Input: part model. Units: mm. Frame: model coordinates. Face numbers are marked on the shaded views. A direction names the side the tool comes from. Coordinates: 2 decimals unless noted, no trailing zeros. Write each loop counter-clockwise with the first axis right and the second up, starting at its lowest first coordinate (ties: lowest second). Pieces come first, ordered by that corner, then holes. Notation, with made-up numbers: M 50.5,26 L 70.5,26 A28 cw 70.5,48 Z; hole C 26,33 d9. An arc over 180 degrees is marked long. Use CSV: the item, a comma, the result in double quotes.
```python
from build123d import *

# Parameters (mm, degrees)
SKETCH_2_W          = 80
SKETCH_2_H          = 82
EXTRUDE_2_DEPTH     = 30
SKETCH_3_R          = 12
CUT_EXTRUDE_1_DEPTH = 65.660652641
CUT_EXTRUDE_2_DEPTH = 65.660652641
HOLE_WIZARD_M4_1_D  = 3.3
HOLE_WIZARD_M4_2_D  = 3.3


with BuildPart() as part:
    # 草图2 → 凸台-拉伸2 (new body)
    with BuildSketch(Plane(origin=(0, 0, 0), x_dir=(0, 0, -1), z_dir=(1, 0, 0))):
        Rectangle(SKETCH_2_W, SKETCH_2_H)
    extrude(amount=EXTRUDE_2_DEPTH)

    # 草图3 → 切除-拉伸1 (cut, through all)
    with BuildSketch(Plane.ZY):
        with Locations((0, 20)):
            Circle(SKETCH_3_R)
    extrude(amount=-CUT_EXTRUDE_1_DEPTH, mode=Mode.SUBTRACT)

    # 草图7 → 切除-拉伸2 (cut, through all)
    with BuildSketch(Plane(origin=(30, 0, 0), x_dir=(0, 0, -1), z_dir=(1, 0, 0))):
        Polygon((-40, 29), (-21, 29), (-21, 4), (21, 4), (21, 29), (40, 29), (40, -41), (-40, -41), align=None)
    extrude(amount=-CUT_EXTRUDE_2_DEPTH, mode=Mode.SUBTRACT)

    # M4 螺纹孔1 (through all)
    with Locations(Plane.ZY):
        with Locations((-11.313708499, 31.313708499), (11.313708499, 8.686291501), (11.313708499, 31.313708499), (16, 20), (-11.313708499, 8.686291501), (-16, 20)):
            Hole(HOLE_WIZARD_M4_1_D / 2)

    # M4 螺纹孔2 (through all)
    with Locations(Plane(origin=(0, 29, 0), x_dir=(-1, 0, 0), z_dir=(0, -1, 0))):
        with Locations((-24, 35), (-6, 35), (-6, 26), (-24, 26), (-6, -35), (-6, -26), (-24, -26), (-24, -35)):
            Hole(HOLE_WIZARD_M4_2_D / 2)


solid = part.part
```
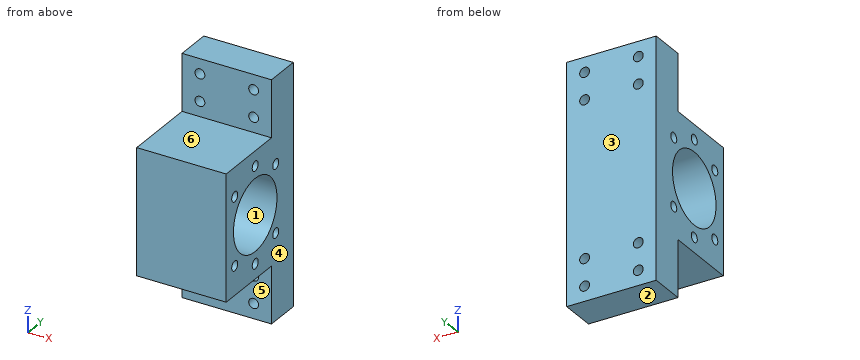
1. Section A-A (z = -16). Return loops of the section in (x, y), then the cut area to 3 significant figures.
Resolved:
outline,"M 0,4 L 30,4 L 30,18.35 L 0,18.35 Z; M 0,21.65 L 30,21.65 L 30,41 L 0,41 Z"
area,"1,010 mm^2"
2. Section D-D (z = -35). Return loops of the section in (x, y).
Resolved:
outline,"M 0,29 L 4.35,29 L 4.35,41 L 0,41 Z; M 7.65,29 L 22.35,29 L 22.35,41 L 7.65,41 Z; M 25.65,29 L 30,29 L 30,41 L 25.65,41 Z"
3. Section B-B (y = 20). Return loops of the section in (x, z), then the cut area to 3 significant figures.
Resolved:
outline,"M 0,-21 L 30,-21 L 30,-17.65 L 0,-17.65 Z; M 0,-14.35 L 30,-14.35 L 30,-12 L 0,-12 Z; M 0,12 L 30,12 L 30,14.35 L 0,14.35 Z; M 0,17.65 L 30,17.65 L 30,21 L 0,21 Z"
area,"342 mm^2"
4. Mould query, pull axis Y, two halves, no side actions, for the marked faces 1, 2 and 3. Classes: pulls with the +Y half, pulls with the -Y half, needs draft (parallel to the pull), parting line crosses it, or undercut.
Resolved:
face 1,"undercut"
face 2,"needs draft"
face 3,"pulls with the +Y half"
5. Material intervals for line 1 (X direction, y = 36.5, z = 35); line 2 (Z direction, x = 24, y = 35.5); line 3 (Y direction, x = 6.25, z = -16), sorted ascending. Write a range as [from, to].
Resolved:
line 1,"x = [0, 4.35], [7.65, 22.35], [25.65, 30]"
line 2,"z = [-40, -36.65], [-33.35, -27.65], [-24.35, 24.35], [27.65, 33.35], [36.65, 40]"
line 3,"y = [4, 18.35], [21.65, 41]"
6. Contact query for flat-ended pins moving along their axis: pin 1 Ø1 at (x, y) = (10, 18) entering from -Z; pin 2 Ø8 at (x, y) = (11.5, 10.5) entering from +Z; pin 3 Ø2 at (y, z) = (33.5, 26) entering from -X; pin 4 Ø4.5 at (x, z) = (24, -26) entering from -Y. Output: stop coordinate, or through.
Resolved:
pin 1,"stops at z = -21"
pin 2,"stops at z = 21"
pin 3,"stops at x = 0"
pin 4,"stops at y = 29"
7. Section C-C (x = 6). State how many separate pieces and enclosed holes the cut face has, then the cut area to 3 significant figures.
Resolved:
separate pieces,"5"
enclosed holes,"7"
area,"1,350 mm^2"
8. Access query for the marked faces 4, 5 and 6. Directions: +Z, -Z, +X, -X, +Y, -Y. A direction counts if a zero-diameter tool reaches every point of the face in a straight line with its end or side. Return the directions, or none.
Resolved:
face 4,"+Z, -Z, +X, +Y, -Y"
face 5,"-Z, +X, -X, -Y"
face 6,"+Z, +X, -X, -Y"
